```python
from build123d import *

# Parameters (mm, degrees)
ESQUISSE1_R                         = 17.9
ESQUISSE1_R_2                       = 15.9
ESQUISSE5_R                         = 16.3
ESQUISSE5_R_2                       = 14.3
BOSS_EXTRU_1_DEPTH                  = 30
BOSS_EXTRU_1_DEPTH_BACK             = 20
BOSS_EXTRU_2_REACH                  = 71.734
BOSS_EXTRU_2_END_RADIUS             = 16.3
ESQUISSE8_R                         = 15.5
ESQUISSE8_R_2                       = 12.5
BOSS_EXTRU_2_DIRECTION_2_REACH      = 71.734
BOSS_EXTRU_2_DIRECTION_2_END_RADIUS = 17.9


with BuildPart() as part:
    # Balayage1: sweep along a path in Esquisse2
    with BuildLine(Plane(origin=(0, 0, 0), x_dir=(0, 0, -1), z_dir=(1, 0, 0))) as balayage1_path:
        Line((-35, 0), (35, 0))
    # Esquisse1 → Balayage1 (sweep)
    with BuildSketch(Plane.XY):
        Circle(ESQUISSE1_R)
        Circle(ESQUISSE1_R_2, mode=Mode.SUBTRACT)
    sweep(path=balayage1_path.line)



with BuildPart() as body_2:
    # Esquisse5 → Boss.-Extru.1 (new, two sides)
    with BuildSketch(Plane(origin=(0, -26.71342567, 0), x_dir=(1, 0, 0), z_dir=(0, 1, 0))) as boss_extru_1_sk:
        with Locations(Location((64.702340676, 0, 0), (0, 0, 270))):
            Circle(ESQUISSE5_R)
        with Locations(Location((64.702340676, 0, 0), (0, 0, 270))):
            Circle(ESQUISSE5_R_2, mode=Mode.SUBTRACT)
    extrude(amount=BOSS_EXTRU_1_DEPTH)
    extrude(boss_extru_1_sk.sketch, amount=-BOSS_EXTRU_1_DEPTH_BACK)


with BuildPart() as part_1:
    add(part.part)

    add(body_2.part)  # Boss.-Extru.2 merges body 2
    # Boss.-Extru.2: up to this cylinder (the profile starts outside it)
    boss_extru_2_end = Plane(origin=(64.702340676, -27.278432, 0), z_dir=(0, 1, 0)) * Cylinder(BOSS_EXTRU_2_END_RADIUS, 177.068, mode=Mode.PRIVATE)
    # Esquisse8 → Boss.-Extru.2 (add, up to the surface)
    with BuildSketch(Plane(origin=(32.351170338, -13.356712835, 0), x_dir=(0, 0, -1), z_dir=(0.9243191525163077, -0.381620366714795, 0)), mode=Mode.PRIVATE) as boss_extru_2_sk1:
        with Locations(Location((0, 0, 0), (0, 0, 90))):
            Circle(ESQUISSE8_R)
        with Locations(Location((0, 0, 0), (0, 0, 90))):
            Circle(ESQUISSE8_R_2, mode=Mode.SUBTRACT)
    boss_extru_2_tool1 = extrude(boss_extru_2_sk1.sketch, amount=BOSS_EXTRU_2_REACH, mode=Mode.PRIVATE) - boss_extru_2_end
    add(boss_extru_2_tool1.solids().sort_by_distance((26.603359, -27.278432, 0))[0])

    # Boss.-Extru.2 direction 2: up to this cylinder (the profile starts outside it)
    boss_extru_2_direction_2_end = Plane(origin=(0, 0, 0), z_dir=(0, 0, 1)) * Cylinder(BOSS_EXTRU_2_DIRECTION_2_END_RADIUS, 180.268, mode=Mode.PRIVATE)
    # Esquisse8 → Boss.-Extru.2 direction 2 (add, up to the surface)
    with BuildSketch(Plane(origin=(32.351170338, -13.356712835, 0), x_dir=(0, 0, -1), z_dir=(0.9243191525163077, -0.381620366714795, 0)), mode=Mode.PRIVATE) as boss_extru_2_direction_2_sk1:
        with Locations(Location((0, 0, 0), (0, 0, 90))):
            Circle(ESQUISSE8_R)
        with Locations(Location((0, 0, 0), (0, 0, 90))):
            Circle(ESQUISSE8_R_2, mode=Mode.SUBTRACT)
    boss_extru_2_direction_2_tool1 = extrude(boss_extru_2_direction_2_sk1.sketch, amount=-BOSS_EXTRU_2_DIRECTION_2_REACH, mode=Mode.PRIVATE) - boss_extru_2_direction_2_end
    add(boss_extru_2_direction_2_tool1.solids().sort_by_distance((26.603359, -27.278432, 0))[0])


solid = part_1.part
```
The listing builds one solid part. Answer for the finished solid, in the listing's coordinates (mm). A direction names the side the tool comes from. Give positions to 0.01 mm unless a question says otherwise; leave off trailing zeros. Loops run counter-clockwise (first coordinate to the right, second up) from the corner with the lowest first, then second, coordinate; pieces in that order, holes last. Notation, with made-up numbers: (71, -6) - (88, -6) arc R25 ccw to (88, 21) - close; hole circle Ø6 at (-15, 83.25). An arc over 180 degrees is marked (long way). Answer as CSV lines item,"result". Start each with the question number.
Item 1: A cutting plane is placed at D-D on y = 5. Count the separate pieces of the cut face and the enclosed holes in it, then the cut area to 3 significant figures.
Item 2: The mould has two halves that part along Y. Classify faces 3 (the face through (16.6, -6.7, -0.2)), 4 (the face through (50, 3.287, 0)), 5 (the face through (-1.4, 16, 35)): +Y half, -Y half, draft (parallel to the pull), parting line (faces both ways), or undercut.
Item 3: For faces 1 (the face through (48.404, -19.795, -0.199)), 2 (the face through (-1.4, 16, -35)), determine the directions among +Z, -Z, +X, -X, +Y, -Y from which every point of the face is accessible in a straight line to the end or side of a thin tool.
Item 4: A cutting plane is placed at C-C on z = -21. Determine the outline of the cut face in (x, y).
Item 5: Each of these flat-tipped pins is pushed along its axis until it touches: pin 1 (5 mm diameter, centred on y = -12.5, z = -7, fed in from +X); pin 2 (12 mm diameter, centred on y = 7.5, z = -20, fed in from -X); pin 3 (12 mm diameter, centred on y = -10, z = 12.5, fed in from -X). Where does it stop, or does it pass through?
Item 6: Find the intervals of material crossed by line 1 (Y direction, x = 0, z = -8); line 2 (X direction, y = -29, z = 0); line 3 (X direction, y = -29, z = -4.5), in increasing order. Write a range as from..to.
Item 7: A cutting plane is placed at B-B on z = -4.5. Determine the outline of the cut face in (x, y).
Item 8: A cutting plane is placed at A-A on x = 0. Determine the outline of the cut face in (y, z).
Found:
1,separate pieces,"2"
1,enclosed holes,"1"
1,area,"434 mm^2"
2,face 3,"undercut"
2,face 4,"+Y half"
2,face 5,"draft"
3,face 1,"none"
3,face 2,"-Z, +X, -X, +Y, -Y"
4,outline,"circle Ø35.8 at (0, 0); hole circle Ø31.8 at (0, 0)"
5,pin 1,"stops at x = 80.37"
5,pin 2,"stops at x = -17.84"
5,pin 3,"stops at x = -17.45"
6,line 1,"y = -17.9..-15.9, 15.9..17.9"
6,line 2,"x = 29.62..37.49, 48.4..50.4, 79..81"
6,line 3,"x = 31.37..39.68, 49.04..51.13, 78.28..80.37"
7,outline,"(3.6, -17.53) - (49.04, -36.29) - (49.04, -46.71) - (51.13, -46.71) - (51.13, 3.29) - (49.04, 3.29) - (49.04, -4.2) - (14.92, 9.89) arc R17.9 ccw (long way) to start; (78.28, -46.71) - (80.37, -46.71) - (80.37, 3.29) - (78.28, 3.29) - close; hole circle Ø31.8 at (0, 0); hole (8.1, -15.96) - (49.04, -32.86) - (49.04, -7.63) - (17, 5.6) arc R17.9 cw to start"
8,outline,"(-17.9, -35) - (-15.9, -35) - (-15.9, 35) - (-17.9, 35) - close; (15.9, -35) - (17.9, -35) - (17.9, 35) - (15.9, 35) - close"
